Autodesk Inventor part; units mm, degrees
ref_plane "YZ Plane" through (0, 0, 0) normal (1, 0, 0) x (0, 1, 0)
ref_plane "XZ Plane" through (0, 0, 0) normal (0, 1, 0) x (-1, 0, 0)
ref_plane "XY Plane" through (0, 0, 0) normal (0, 0, 1) x (1, 0, 0)
sketch "Sketch1" plane through (0, 0, 0) normal (0, 1, 0) x (-1, 0, 0)
  circle A0 centre (0, 0) radius 1.97
  circle A1 centre (0, 0) radius 3.5
  line L0 (0.866, -1.5) -> (-0.866, -1.5)
  line L1 (-0.866, -1.5) -> (-1.7321, 0)
  line L2 (-1.7321, 0) -> (-0.866, 1.5)
  line L3 (-0.866, 1.5) -> (0.866, 1.5)
  line L4 (0.866, 1.5) -> (1.7321, 0)
  line L5 (1.7321, 0) -> (0.866, -1.5)
  dimension "d0" = 3.94
  dimension "d1" = 7
  dimension "d8" = 3
extrude "Extrusion1" add sketch "Sketch1" along normal blind 4 contours A0 | A1 | L0 L1 L2 L3 L4 L5
extrude "Extrusion2" add sketch "Sketch1" against normal blind 20 contours A0 | L0 L1 L2 L3 L4 L5
extrude "Extrusion3" cut sketch "Sketch1" against normal blind 3 from surface at 4 contours L0 L1 L2 L3 L4 L5
fillet "Fillet1" radius 0.5 1 edges at (3.5, 4, 0)
thread "Thread2"
equation "\"d4\" = length"
equation "\"length\" = 20"
properties part number "M4x20"
Read the model definition and answer for the solid it produces. Units are mm, in the model's axes. A direction names the side the tool comes from. Give positions to 0.01 mm unless a question says otherwise; leave off trailing zeros. Write each loop counter-clockwise with the first axis right and the second up, starting at its lowest first coordinate (ties: lowest second). Pieces come first, ordered by that corner, then holes. Notation, with made-up numbers: (88.25, -20.75) -> (130.25, -20.75) arc R10 cw to (130.25, -6.75) -> close; hole circle Ø8 at (20.25, 44). An arc over 180 degrees is marked (long way). Answer as a JSON object with one key per item and string values. Group by question number.
1) Consider L1, parallel to Y at x = 2.25, z = 0.25; L2, parallel to Y at x = 1, z = 0; L3, parallel to X at y = 2.5, z = 1.25. Determine where each line is inside the solid, lowest interval first. Write a range as from..to.
2) Find section B-B (x = 0). Write down the section's boundary in (y, z).
3) A tool of negligible diameter and unlimited length cuts with its end or side. For faces 1 (the flat face through (1.305, 2.521, 0.74)), 2 (the flat face through (-2, 0, -2)), 3 (the flat face through (0, -20, 0)), from which of +Z, -Z, +X, -X, +Y, -Y can it reach the whole face along a straight path? Write none if from no direction.
4) This flat-tipped pin is pushed along its axis until it touches: P1, Ø1.5, axis at x = 0, y = -6.5, coming from the -Z side. Where does it stop, or does it pass through?
5) Find section A-A (y = 2.5). Write down the section's boundary in (x, z), and give its area (3 significant figures).
6) The mould has two halves that part along Z. Classify faces 4 (the cylindrical face through (0.427, -9.86, -1.923)), 5 (the flat face through (-1.305, 2.521, -0.74)), 6 (the flat face through (1.293, 2.521, -0.76)), 7 (the flat face through (-1.3, 4, -1.3)): +Z half, -Z half, draft (parallel to the pull), parting line (faces both ways), or undercut.
7) Find section C-C (y = -14.75). Write down the section's boundary in (x, z), and give its area (3 significant figures).
Values follow:
{
 "1": {"L1": "y = 0..4", "L2": "y = -20..1", "L3": "x = -3.27..-1.01, 1.01..3.27"},
 "2": {"outline": "(-20, -1.97) -> (0, -1.97) -> (0, -3.5) -> (3.5, -3.5) arc R0.5 ccw to (4, -3) -> (4, -1.5) -> (1, -1.5) -> (1, 1.5) -> (4, 1.5) -> (4, 3) arc R0.5 ccw to (3.5, 3.5) -> (0, 3.5) -> (0, 1.97) -> (-20, 1.97) -> close"},
 "3": {"face 1": "+Y", "face 2": "-Y", "face 3": "+Z, -Z, +X, -X, -Y"},
 "4": {"P1": "stops at z = -1.97"},
 "5": {"outline": "circle Ø7 at (0, 0); hole (-1.73, 0) -> (-0.87, -1.5) -> (0.87, -1.5) -> (1.73, 0) -> (0.87, 1.5) -> (-0.87, 1.5) -> close", "area": "30.7 mm2"},
 "6": {"face 4": "parting line", "face 5": "undercut", "face 6": "undercut", "face 7": "draft"},
 "7": {"outline": "circle Ø3.94 at (0, 0)", "area": "12.2 mm2"}
}
